Design review of the part built by this model. Coordinates are the model's own, in mm. Coordinates: 2 decimals unless noted, no trailing zeros. Order: outer loops, then holes, each group sorted by start corner. A loop starts at its lowest first (then second) coordinate and runs counter-clockwise, first axis right, second up. Notation, with made-up numbers: M 55,-27 L 96,-27 A18 cw 96,4 Z; hole C -18,82.25 d7. An arc over 180 degrees is marked long. Answer in a Markdown table with one row per item.
from build123d import *

# Parameters (mm, degrees)
SKETCH2_W           = 70
SKETCH2_H           = 70
BOSS_EXTRUDE1_DEPTH = 20
SKETCH3_R           = 2.05
CUT_EXTRUDE1_DEPTH  = 54.38539126
SKETCH4_R           = 21.658851084
CUT_EXTRUDE2_DEPTH  = 54.38539126


with BuildPart() as part:
    # Sketch2 → Boss-Extrude1 (new body)
    with BuildSketch(Plane(origin=(0, 0, 0), x_dir=(1, 0, 0), z_dir=(0, 1, 0))):
        Rectangle(SKETCH2_W, SKETCH2_H)
    extrude(amount=-BOSS_EXTRUDE1_DEPTH)

    # Sketch1 → Cut-Revolve1 (revolve, cut)
    with BuildSketch(Plane.XY, mode=Mode.PRIVATE) as cut_revolve1_sk:
        with BuildLine():
            Line((0, -17.2), (0, 0))
            Line((0, 0), (21.241684944, 0))
            Line((21.241684944, 0), (21.158851084, -0.511526958))
            add(Edge.make_bspline(
                [(0, -17.2), (0.530678283, -17.2), (1.61157482, -17.183508716), (3.615531125, -17.08588663), (5.944127269, -16.844919371), (8.44843367, -16.370131279), (11.442656399, -15.492934033), (14.579654851, -13.93724298), (17.382164488, -11.402739011), (19.199009229, -8.500896664), (20.23569058, -5.583194157), (20.706490619, -3.313387562), (20.981886079, -1.635929169), (21.096876841, -0.894238762), (21.158851084, -0.511526958)],
                knots=[0, 0, 0, 0, 0.03125, 0.0625, 0.125, 0.1875, 0.25, 0.375, 0.5, 0.625, 0.75, 0.875, 0.9375, 1, 1, 1, 1], degree=3))
        make_face()
    revolve(cut_revolve1_sk.sketch.rotate(Axis((0, -17.2, 0), (0, 1, 0)), 90), axis=Axis((0, -17.2, 0), (0, 1, 0)), mode=Mode.SUBTRACT)

    # Sketch3 → Cut-Extrude1 (cut, through all)
    with BuildSketch(Plane(origin=(0, 0, 0), x_dir=(1, 0, 0), z_dir=(0, 1, 0))):
        with Locations(Location((-19, 19, 0), (0, 0, 270))):
            Circle(SKETCH3_R)
        with Locations(Location((19, -19, 0), (0, 0, 90))):
            Circle(SKETCH3_R)
        with Locations(Location((-19, -19, 0), (0, 0, 90))):
            Circle(SKETCH3_R)
        with Locations(Location((19, 19, 0), (0, 0, 270))):
            Circle(SKETCH3_R)
    extrude(amount=-CUT_EXTRUDE1_DEPTH, mode=Mode.SUBTRACT)

    # Sketch4 → Cut-Extrude2 (cut, through all)
    with BuildSketch(Plane(origin=(0, 0, 0), x_dir=(1, 0, 0), z_dir=(0, 1, 0))):
        with Locations(Location((0, 0, 0), (0, 0, 270))):
            Circle(SKETCH4_R)
    extrude(amount=-CUT_EXTRUDE2_DEPTH, mode=Mode.SUBTRACT)


solid = part.part
(1) Add section C-C, the plane y = -10. Give the boundary of the cut face in (x, z).
Return value:
| item | result |
|---|---|
| outline | M -35,-35 L 35,-35 L 35,35 L -35,35 Z; hole C 0,0 d43.32; hole C -19,-19 d4.1; hole C -19,19 d4.1; hole C 19,-19 d4.1; hole C 19,19 d4.1 |
(2) Add section B-B, the plane z = -5. Give the boundary of the cut face in (x, y).
Return value:
| item | result |
|---|---|
| outline | M -35,-20 L -21.07,-20 L -21.07,0 L -35,0 Z; M 21.07,-20 L 35,-20 L 35,0 L 21.07,0 Z |
(3) Draft analysis for pull direction Z (two halves, no side actions). For faces 1 (the flat face through (0, -10, 35)), 2 (the flat face through (-16, -20, -16)), 3 (the cylindrical face through (17.6, -9.9, 20.5)), state which applies: pulls with the +Z half, pulls with the -Z half, needs draft (parallel to the pull), parting line crosses it, or undercut.
Return value:
| item | result |
|---|---|
| face 1 | pulls with the +Z half |
| face 2 | needs draft |
| face 3 | undercut |
(4) Add section A-A, the plane x = 0. Give the boundary of the cut face in (y, z), and give its area (3 significant figures).
Return value:
| item | result |
|---|---|
| outline | M -20,-35 L 0,-35 L 0,-21.66 L -20,-21.66 Z; M -20,21.66 L 0,21.66 L 0,35 L -20,35 Z |
| area | 534 mm2 |
(5) For line 1 along X through (y, z) = (-10.5, 0); line 2 along X through (y, z) = (-10.25, -19); line 3 along Z through (x, y) = (-3, -1.5), list the stretches that pass through material, from the lowest coordinate up. Write a range as from..to.
Return value:
| item | result |
|---|---|
| line 1 | x = -35..-21.66, 21.66..35 |
| line 2 | x = -35..-21.05, -16.95..-10.4, 10.4..16.95, 21.05..35 |
| line 3 | z = -35..-21.45, 21.45..35 |
(6) Add section D-D, the plane z = 18.5. Give the boundary of the cut face in (x, y), and give its area (3 significant figures).
Return value:
| item | result |
|---|---|
| outline | M -35,-20 L -20.99,-20 L -20.99,0 L -35,0 Z; M -17.01,-20 L -11.26,-20 L -11.26,0 L -17.01,0 Z; M 11.26,-20 L 17.01,-20 L 17.01,0 L 11.26,0 Z; M 20.99,-20 L 35,-20 L 35,0 L 20.99,0 Z |
| area | 790 mm2 |
